Model file for the job. Use its own axes, mm. Give positions to 0.01 mm unless a question says otherwise; leave off trailing zeros. Loops run counter-clockwise (first coordinate to the right, second up) from the corner with the lowest first, then second, coordinate; pieces in that order, holes last. Notation, with made-up numbers: (70.25, 30) - (118.25, 30) arc R17 ccw to (118.25, 51) - close; hole circle Ø11 at (56, 48.5). An arc over 180 degrees is marked (long way). Use a Markdown table: item, result.
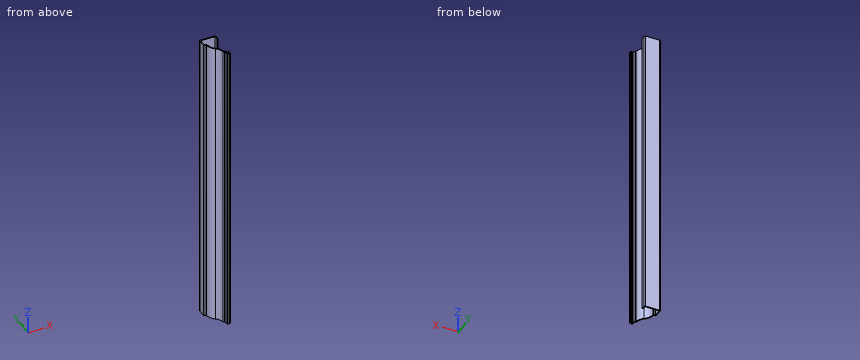
from build123d import *

# Parameters (mm, degrees)
EXTRUDE_THIN1_DEPTH = 412.75
FILLET1_R           = 1.27


with BuildPart() as part:
    # Sketch1 → Extrude-Thin1 (new body)
    with BuildSketch(Plane.XY):
        with BuildLine():
            Line((0, 4.7625), (0, 0))
            Line((0, 0), (-4.7625, 0))
            Line((-4.7625, 0), (-4.7625, 5.55625))
            Line((-4.7625, 5.55625), (-7.14375, 5.55625))
            ThreePointArc((-7.14375, 5.55625), (-8.548737384, 11.551507081), (-12.471121185, 16.298295714))
            ThreePointArc((-12.471121185, 16.298295714), (-17.097302988, 21.720310148), (-19.05, 28.575))
            Line((-19.05, 28.575), (-22.225, 28.575))
            Line((-22.225, 28.575), (-22.225, 41.275))
            Line((-22.225, 41.275), (0, 40.878125))
            Line((0, 40.878125), (0, 34.528125))
            Line((0, 34.528125), (-1.27, 34.528125))
            Line((-1.27, 34.528125), (-1.27, 39.6306011))
            Line((-1.27, 39.6306011), (-20.955, 39.982118957))
            Line((-20.955, 39.982118957), (-20.955, 29.845))
            Line((-20.955, 29.845), (-17.811850471, 29.845))
            ThreePointArc((-17.811850471, 29.845), (-16.248920172, 22.850151694), (-11.702520826, 17.309311781))
            ThreePointArc((-11.702520826, 17.309311781), (-7.705625486, 12.679096033), (-5.928475081, 6.82625))
            Line((-5.928475081, 6.82625), (-3.4925, 6.82625))
            Line((-3.4925, 6.82625), (-3.4925, 1.27))
            Line((-3.4925, 1.27), (-1.27, 1.27))
            Line((-1.27, 1.27), (-1.27, 4.7625))
            Line((-1.27, 4.7625), (0, 4.7625))
        make_face()
    extrude(amount=-EXTRUDE_THIN1_DEPTH)

    # Fillet1
    fillet1_edges = [part.edges().sort_by_distance(p)[0] for p in [
        (-17.811850471, 29.845, -206.375),
        (-3.4925, 6.82625, -206.375),
        (0, 0, -206.375),
        (-4.7625, 0, -206.375),
        (-7.14375, 5.55625, -206.375),
        (-22.225, 28.575, -206.375),
        (-22.225, 41.275, -206.375),
        (0, 40.878125, -206.375),
    ]]
    fillet(fillet1_edges, radius=FILLET1_R)


solid = part.part
(1) Slice it at B-B, the plane y = 22. Write the cut outline in (x, z), plus the area to 3 significant figures.
Computed:
| item | result |
|---|---|
| outline | (-17.24, -412.75) - (-15.8, -412.75) - (-15.8, 0) - (-17.24, 0) - close |
| area | 595 mm² |
(2) Drill centre lines: probe 1 along X at (y, z) = (3, -238); probe 2 along Y at (x, z) = (-2.75, -45); probe 3 along Y at (x, z) = (-5.5, -232). Where is each one in solid material? Low to high. Write a range as [from, to].
Computed:
| item | result |
|---|---|
| probe 1 | [-4.76, -3.49], [-1.27, 0] |
| probe 2 | [0, 1.27], [39.66, 40.93] |
| probe 3 | [5.56, 6.83], [39.71, 40.98] |
(3) Pin check, flat tips, straight feed: P1, Ø0.6, axis at x = -5.5, z = -259, coming from the +Y side; P2, Ø2, axis at y = 4, z = -145.5, coming from the -X side; P3, Ø5, axis at x = -9.5, y = 12.5, coming from the +Z side; P4, Ø6, axis at x = -7.5, z = -291.5, coming from the +Y side. Stop position of each tip, or through.
Computed:
| item | result |
|---|---|
| P1 | y = 40.98 |
| P2 | x = -4.76 |
| P3 | z = 0 |
| P4 | y = 41.07 |
